Autodesk Inventor part; units mm, degrees
ref_plane "dia1_XY" through (0, 2.3749, 0) normal (1, 0, 0) x (0, 0, -1)
ref_plane "dia1_YZ" through (0, 2.3749, 0) normal (0, 0, -1) x (0, 1, 0)
ref_plane "dia1_ZX" through (0, 2.3749, 0) normal (0, 1, 0) x (1, 0, 0)
sketch "Sketch_1" plane through (0, 0, 0) normal (0, 0, 1) x (1, 0, 0)
  line L0 (95.9866, 0) -> (0, 0)
  line L1 (0, 0) -> (0, 2.3749)
  line L2 (0, 2.3749) -> (80.1624, 2.3749)
  line L3 (80.1624, 2.3749) -> (80.1624, 7.22)
  line L4 (80.1624, 7.22) -> (95.9866, 7.22)
  line L5 (95.9866, 7.22) -> (95.9866, 0)
  line L6 (95.9866, 0) -> (0, 0)
revolve "Revolution1" add sketch "Sketch_1" angle 360 about axis through (95.9866, 0, 0) along (1, 0, 0)
sketch "Sketch_3" plane through (0, 0, 0) normal (0, 0, 1) x (1, 0, 0)
  line L0 (0, 0) -> (-12.7, 0)
  line L1 (-12.7, 0) -> (-12.7, 1.9406)
  line L2 (-12.7, 1.9406) -> (-12.2276, 2.413)
  line L3 (-12.2276, 2.413) -> (0, 2.413)
  line L4 (0, 2.413) -> (0, 0)
  line L5 (0, 0) -> (-12.7, 0)
revolve "Revolution2" add sketch "Sketch_3" angle 360 about axis through (0, 0, 0) along (1, 0, 0)
thread "Thread1"
sketch "Sketch_30" plane through (0, 0, 0) normal (0, 0, 1) x (1, 0, 0)
  line L0 (0, 0) -> (-0.254, 0)
  line L1 (-0.254, 2.159) -> (0, 2.159)
  line L2 (0, 2.159) -> (0, 2.667)
  line L3 (0, 2.667) -> (-0.254, 2.667)
  line L4 (-0.254, 2.667) -> (-0.254, 2.159)
revolve "Revolution3" cut sketch "Sketch_30" angle 360 about axis through (0, 0, 0) along (1, 0, 0)
ref_plane "dia1_XY" through (0, 2.3749, 0) normal (1, 0, 0) x (0, 0, -1)
ref_plane "dia1_YZ" through (0, 2.3749, 0) normal (0, 0, -1) x (0, 1, 0)
ref_plane "dia1_ZX" through (0, 2.3749, 0) normal (0, 1, 0) x (1, 0, 0)
ref_plane "dia12_XY" through (0, 0, 7.8105) normal (1, 0, 0) x (0, 0, -1)
ref_plane "dia12_YZ" through (0, 0, 7.8105) normal (0, 0, -1) x (0, 1, 0)
ref_plane "dia12_ZX" through (0, 0, 7.8105) normal (0, 1, 0) x (1, 0, 0)
ref_plane "dia2_XY" through (0, -2.3749, 0) normal (1, 0, 0) x (0, 0, -1)
ref_plane "dia2_YZ" through (0, -2.3749, 0) normal (0, 0, -1) x (0, 1, 0)
ref_plane "dia2_ZX" through (0, -2.3749, 0) normal (0, 1, 0) x (1, 0, 0)
ref_plane "dia22_XY" through (0, 0, -7.8105) normal (1, 0, 0) x (0, 0, -1)
ref_plane "dia22_YZ" through (0, 0, -7.8105) normal (0, 0, -1) x (0, 1, 0)
ref_plane "dia22_ZX" through (0, 0, -7.8105) normal (0, 1, 0) x (1, 0, 0)
ref_plane "rl1_XY" through (-12.7, 0, 0) normal (1, 0, 0) x (0, 0, -1)
ref_plane "rl1_YZ" through (-12.7, 0, 0) normal (0, 0, -1) x (0, 1, 0)
ref_plane "rl1_ZX" through (-12.7, 0, 0) normal (0, 1, 0) x (1, 0, 0)
ref_plane "rl2_XY" through (0, 0, 0) normal (1, 0, 0) x (0, 0, -1)
ref_plane "rl2_YZ" through (0, 0, 0) normal (0, 0, -1) x (0, 1, 0)
ref_plane "rl2_ZX" through (0, 0, 0) normal (0, 1, 0) x (1, 0, 0)
ref_plane "rod_cp_XY" through (0, 0, 0) normal (1, 0, 0) x (0, 0, -1)
ref_plane "rod_cp_YZ" through (0, 0, 0) normal (0, 0, -1) x (0, 1, 0)
ref_plane "rod_cp_ZX" through (0, 0, 0) normal (0, 1, 0) x (1, 0, 0)
ref_plane "thd1_XY" through (-12.7, 2.413, 0) normal (1, 0, 0) x (0, 0, -1)
ref_plane "thd1_YZ" through (-12.7, 2.413, 0) normal (0, 0, -1) x (0, 1, 0)
ref_plane "thd1_ZX" through (-12.7, 2.413, 0) normal (0, 1, 0) x (1, 0, 0)
ref_plane "thd2_XY" through (-12.7, -2.413, 0) normal (1, 0, 0) x (0, 0, -1)
ref_plane "thd2_YZ" through (-12.7, -2.413, 0) normal (0, 0, -1) x (0, 1, 0)
ref_plane "thd2_ZX" through (-12.7, -2.413, 0) normal (0, 1, 0) x (1, 0, 0)
ref_plane "to_rod_clevis_XY" through (-12.7, 0, 0) normal (1, 0, 0) x (0, 0, -1)
ref_plane "to_rod_clevis_YZ" through (-12.7, 0, 0) normal (0, 0, -1) x (0, 1, 0)
ref_plane "to_rod_clevis_ZX" through (-12.7, 0, 0) normal (0, 1, 0) x (1, 0, 0)
properties part number "022-DXP0000_rod"
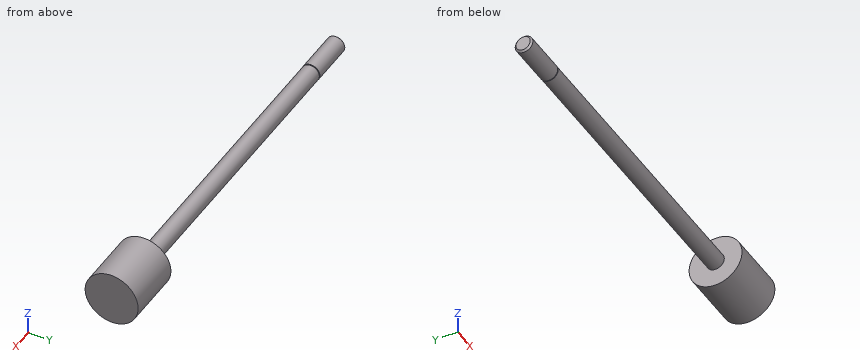
For this review, take the finished solid that the model builds, in its own axes (mm). Give positions to 0.01 mm unless a question says otherwise; leave off trailing zeros. Loops run counter-clockwise (first coordinate to the right, second up) from the corner with the lowest first, then second, coordinate; pieces in that order, holes last. Notation, with made-up numbers: M -14,34 L 15,34 A19 cw 15,51 Z; hole C 26.5,88.5 d1. An arc over 180 degrees is marked long. Answer as a JSON object with one key per item and string values. Group by question number.
Q1. Add section C-C on x = 64.5. Give the boundary of the cut face in (y, z), and give its area (3 significant figures).
Q2. For probe 1 along X at (y, z) = (2.5, -0.25); probe 2 along Z at (x, y) = (50, -1); probe 3 along X at (y, z) = (2.25, 0), list the stretches that pass through material, from the lowest coordinate up. Write a range as [from, to].
Q3. Add section A-A on z = 0. Give the boundary of the cut face in (x, y).
Q4. Add section D-D on x = 85. Give the boundary of the cut face in (y, z), and give its area (3 significant figures).
Q5. Insertion check: P1, Ø4, axis at x = 39.5, z = 4, coming from the +Y side; P2, Ø8, axis at x = 29.5, z = -3, coming from the -Y side; P3, Ø4, axis at y = 5.5, z = 1.5, coming from the -X side. Each pin has a flat end and moves straight along its axis. Give the tip position at first contact, or say it passes through.
Checked values:
{
 "1": {"outline": "C 0,0 d4.75", "area": "17.7 mm²"},
 "2": {"probe 1": "[80.16, 95.99]", "probe 2": "[-2.15, 2.15]", "probe 3": "[-12.39, -0.25], [0, 95.99]"},
 "3": {"outline": "M -12.7,-1.94 L -12.23,-2.41 L -0.25,-2.41 L -0.25,-2.16 L 0,-2.16 L 0,-2.37 L 80.16,-2.37 L 80.16,-7.22 L 95.99,-7.22 L 95.99,7.22 L 80.16,7.22 L 80.16,2.37 L 0,2.37 L 0,2.16 L -0.25,2.16 L -0.25,2.41 L -12.23,2.41 L -12.7,1.94 Z"},
 "4": {"outline": "C 0,0 d14.44", "area": "164 mm²"},
 "5": {"P1": "y = 1.28", "P2": "y = -2.37", "P3": "x = 80.16"}
}
